Work out the finished part from the listing and answer in its coordinate system (mm). A direction names the side the tool comes from. Round coordinates to 2 decimals unless told otherwise and drop trailing zeros. Loops run counter-clockwise (first coordinate to the right, second up) from the corner with the lowest first, then second, coordinate; pieces in that order, holes last.
from build123d import *

# Parameters (mm, degrees)
F1_DEPTH = 3.5
F3_DEPTH = 59.89472
F4_W     = 42.426407
F4_H     = 3.5
F5_DEPTH = 25.9868
F6_W     = 42.426407
F6_H     = 3.5
F7_DEPTH = 37.73951


with BuildPart() as f1:
    # F0 (on Top) → F1 (new body)
    with BuildSketch(Plane.XY):
        Polygon((-30, 0), (0, 0), (30, 0), (30, 40), (0, 70), (-30, 40), align=None)
        Polygon((26, 4), (-26, 4), (-26, 38.343146), (-12.171573, 52.171573), (0, 64.343146), (26, 38.343146), align=None, mode=Mode.SUBTRACT)
    extrude(amount=F1_DEPTH)

    # F2 (on face) → F3 (join)
    with BuildSketch(Plane(origin=(0, 4, 0), x_dir=(-1, 0, 0), z_dir=(0, 1, 0))):
        Polygon((26, 0), (26, 1), (21.27, 3), (21.27, 1), (16.54, 3), (16.54, 1), (11.81, 3), (11.81, 1), (7.08, 3), (7.08, 1), (2.35, 3), (2.35, 1), (-2.38, 3), (-2.38, 1), (-7.11, 3), (-7.11, 1), (-11.84, 3), (-11.84, 1), (-16.57, 3), (-16.57, 1), (-21.3, 3), (-21.3, 1), (-26, 3), (-26, 0), align=None)
    extrude(amount=F3_DEPTH)

    # F4 (on face) → F5 (cut)
    with BuildSketch(Plane(origin=(35, 35, 0), x_dir=(-0.707107, 0.707107, 0), z_dir=(0.707107, 0.707107, 0))):
        with Locations((28.284271, 1.75)):
            Rectangle(F4_W, F4_H)
    extrude(amount=F5_DEPTH, mode=Mode.SUBTRACT)

    # F6 (on face) → F7 (cut)
    with BuildSketch(Plane(origin=(-35, 35, 0), x_dir=(-0.707107, -0.707107, 0), z_dir=(-0.707107, 0.707107, 0))):
        with Locations((-28.284271, 1.75)):
            Rectangle(F6_W, F6_H)
    extrude(amount=F7_DEPTH, mode=Mode.SUBTRACT)


solid = f1.part
Item 1: Straight lines are drawn through the part: line 1 (Y direction, x = 6.5, z = 3.1); line 2 (Y direction, x = 4, z = 2.95); line 3 (Z direction, x = -9, y = 46). For each, find the intervals that lie inside material, in ascending order.
Item 2: Section B-B, the plane x = 15 is taken. Give the vertices of the cut face in (y, z), plus the area to 3 significant figures.
Item 3: Section A-A, the plane y = 25.5 is taken. Give the vertices of the cut face in (x, z).
Item 4: For faces 5 (the face through (-30, 20, 2)), 6 (the face through (-14.208, 27.927, 1.986)), determine the directions among +Z, -Z, +X, -X, +Y, -Y from which every point of the face is accessible in a straight line to the end or side of a thin tool.
Item 5: Determine the mould class of faces 1 (the face through (-20, 46, 3.5)), 2 (the face through (16.57, 26, 2)), 3 (the face through (15, 55, 2)), 4 (the face through (-0.018, 33.528, 1.986)) for opening direction Y: pulls with the +Y half, pulls with the -Y half, needs draft (parallel to the pull), parting line crosses it, or undercut.
Item 6: Each of these flat-tipped pins is pushed along its axis until it touches: P1, Ø1.5, axis at x = 21.5, z = 3, coming from the +Y side; P2, Ø1, axis at x = 17.5, y = 14.5, coming from the +Z side; P3, Ø0.8, axis at x = -9, z = 2, coming from the +Y side. Where does it stop, or does it pass through?
Item 7: Section C-C, the plane x = 24 is taken. Give the vertices of the cut face in (y, z), plus the area to 3 significant figures.
Answer below:
1. line 1: y = 0 to 4, 57.84 to 63.5
1. line 2: y = 0 to 4, 60.34 to 66
1. line 3: z = 0 to 2.19
2. outline: (0, 0) - (55, 0) - (55, 3.5) - (49.34, 3.5) - (49.34, 2.34) - (4, 2.34) - (4, 3.5) - (0, 3.5) - close
2. area: 140 mm2
3. outline: (-30, 0) - (30, 0) - (30, 3.5) - (26, 3.5) - (26, 3) - (21.3, 1) - (21.3, 3) - (16.57, 1) - (16.57, 3) - (11.84, 1) - (11.84, 3) - (7.11, 1) - (7.11, 3) - (2.38, 1) - (2.38, 3) - (-2.35, 1) - (-2.35, 3) - (-7.08, 1) - (-7.08, 3) - (-11.81, 1) - (-11.81, 3) - (-16.54, 1) - (-16.54, 3) - (-21.27, 1) - (-21.27, 3) - (-26, 1) - (-26, 3.5) - (-30, 3.5) - close
4. face 5: +Z, -Z, -X, +Y, -Y
4. face 6: +Z
5. face 1: needs draft
5. face 2: undercut
5. face 3: pulls with the +Y half
5. face 4: undercut
6. P1: stops at y = 49.25
6. P2: stops at z = 1.6
6. P3: stops at y = 61.4
7. outline: (0, 0) - (46, 0) - (46, 3.5) - (40.34, 3.5) - (40.34, 2.15) - (4, 2.15) - (4, 3.5) - (0, 3.5) - close
7. area: 112 mm2
